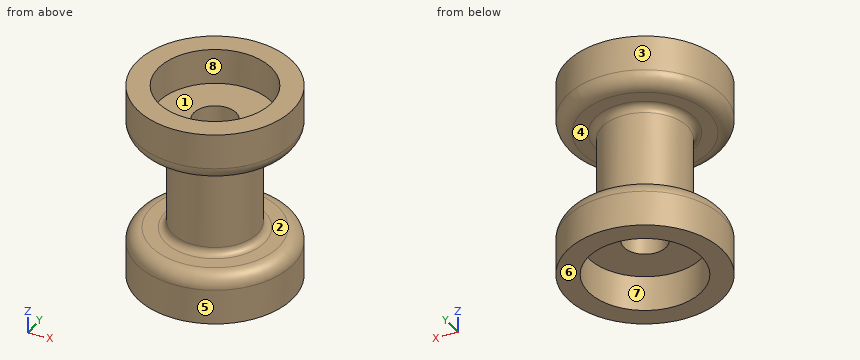
```python
from build123d import *


with BuildPart() as part:
    # Esboço1 → Revolução1 (revolve)
    with BuildSketch(Plane(origin=(0, 0, 0), x_dir=(0, 0, -1), z_dir=(1, 0, 0))):
        with BuildLine():
            Line((0, 8), (0, 11))
            Line((0, 11), (5, 11))
            ThreePointArc((5, 11), (6.414213562, 10.414213562), (7, 9))
            Line((7, 9), (7, 7))
            ThreePointArc((7, 7), (7.292893219, 6.292893219), (8, 6))
            Line((8, 6), (20, 6))
            ThreePointArc((20, 6), (20.707106781, 6.292893219), (21, 7))
            Line((21, 7), (21, 9))
            ThreePointArc((21, 9), (21.585786438, 10.414213562), (23, 11))
            Line((23, 11), (28, 11))
            Line((28, 11), (28, 8))
            Line((28, 8), (23, 8))
            Line((23, 8), (23, 3))
            Line((23, 3), (5, 3))
            Line((5, 3), (5, 8))
            Line((5, 8), (0, 8))
        make_face()
    revolve(axis=Axis((0, 0, 0), (0, 0, -1)))


solid = part.part
```
CAD build for the part. Positions are in the model's coordinates, mm. Face numbers are marked on the shaded views. A direction names the side the tool comes from. Give positions to 0.01 mm unless a question says otherwise; leave off trailing zeros. Loops run counter-clockwise (first coordinate to the right, second up) from the corner with the lowest first, then second, coordinate; pieces in that order, holes last. Notation, with made-up numbers: M -25,-16 L 29,-16 A7 ccw 29,-4 Z; hole C 65.25,5 d4. An arc over 180 degrees is marked long. Use one line per item in the form item = value.
Item 1: Flat gauge pins, fed straight in: pin 1 (4 mm diameter, centred on x = 3.5, y = 3, fed in from +Z); pin 2 (1.5 mm diameter, centred on x = -7.5, z = -6.5, fed in from +Y); pin 3 (9 mm diameter, centred on x = 1.5, y = 1, fed in from -Z). Where does each tip first touch, or does it go through?
Determined:
pin_1 = -5
pin_2 = 8.19
pin_3 = -23
Item 2: Slice it at D-D (z = -18.5). List the corners of the cut face in (x, y), plus the area to 3 significant figures.
Determined:
outline = C 0,0 d12; hole C 0,0 d6
area = 84.8 mm2
Item 3: Two-plate mould, pull along Y, no slides. Class the marked faces 1, 2 and 3: pulls with the +Y half, pulls with the -Y half, needs draft (parallel to the pull), parting line crosses it, or undercut.
Determined:
face_1 = undercut
face_2 = needs draft
face_3 = parting line crosses it
Item 4: Which spindle directions (+Z, -Z, +X, -X, +Y, -Y) get a long thin tool onto all of the face, cutting with end or side? Do the marked faces 4, 5, 6, 7 and 8. Say none if no direction does.
Determined:
face_4 = none
face_5 = +Z, -Z
face_6 = -Z, +X, -X, +Y, -Y
face_7 = -Z
face_8 = +Z
Item 5: Slice it at C-C (z = -3.25). List the corners of the cut face in (x, y).
Determined:
outline = C 0,0 d22; hole C 0,0 d16
Item 6: Drill centre lines: probe 1 along X at (y, z) = (0, -25.4); probe 2 along Z at (x, y) = (-3.5, 8); probe 3 along X at (y, z) = (0, -19.5). Where is each one in solid material? Low to high. Write a range as from..to.
Determined:
probe_1 = -11..-8, 8..11
probe_2 = -28..-21, -7..0
probe_3 = -6..-3, 3..6
